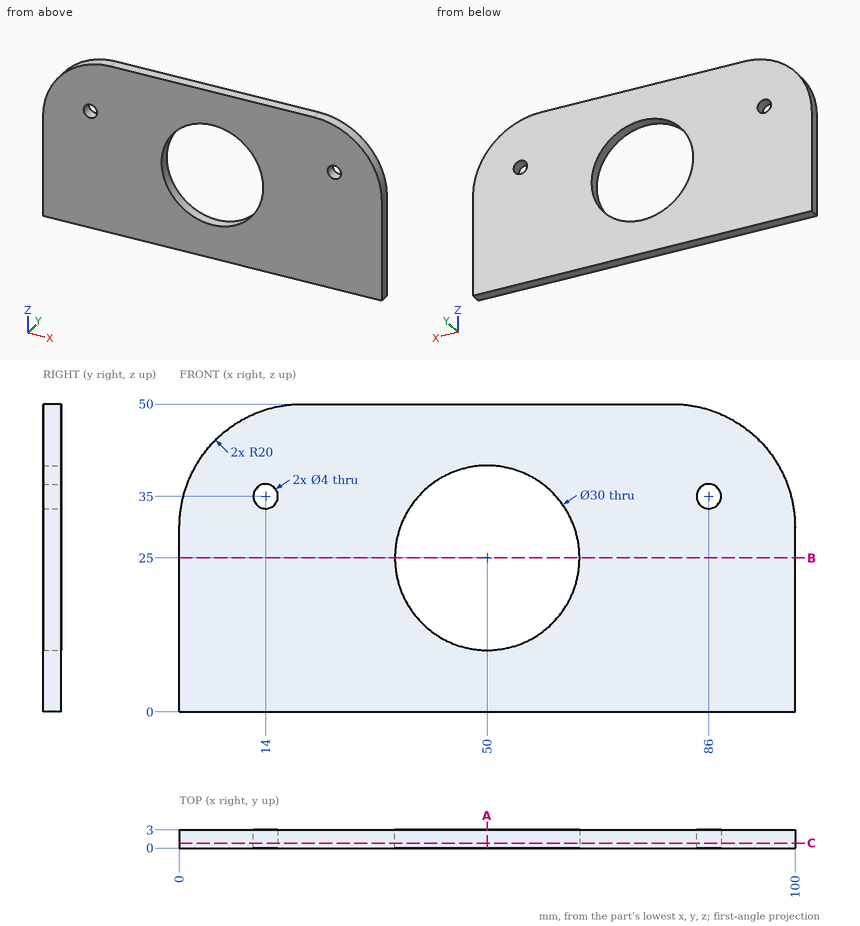
Source: three-view drawing plus pictorial views. Frame: mm from the lowest corner of the part. Round coordinates to 2 decimals unless told otherwise and drop trailing zeros. Order: outer loops, then holes, each group sorted by start corner. A loop starts at its lowest first (then second) coordinate and runs counter-clockwise, first axis right, second up. Notation, with made-up numbers: (-12.5, 33) - (8.5, 33) arc R22 ccw to (8.5, 58) - close; hole circle Ø4 at (-26.5, 72). An arc over 180 degrees is marked (long way). Write each question's results on one line, items separated by ' | '.
Item 1: First-contact query: pin 1 Ø2.5 at (x, z) = (86, 35) entering from -Y. Flat tip, straight axial feed; report the tip coordinate or a pass-through.
Completed:
pin 1: through
Item 2: Section B-B, the plane z = 25. Return the cut outline in (x, y), and give its area (3 significant figures).
Completed:
outline: (0, 0) - (35, 0) - (35, 3) - (0, 3) - close; (65, 0) - (100, 0) - (100, 3) - (65, 3) - close | area: 210 mm^2
Item 3: Section C-C, the plane y = 0.85. Return the cut outline in (x, z), and give its area (3 significant figures).
Completed:
outline: (0, 0) - (100, 0) - (100, 30) arc R20 ccw to (80, 50) - (20, 50) arc R20 ccw to (0, 30) - close; hole circle Ø4 at (14, 35); hole circle Ø30 at (50, 25); hole circle Ø4 at (86, 35) | area: 4,100 mm^2
Item 4: Section A-A, the plane x = 50. Return the cut outline in (y, z), and give its area (3 significant figures).
Completed:
outline: (0, 0) - (3, 0) - (3, 10) - (0, 10) - close; (0, 40) - (3, 40) - (3, 50) - (0, 50) - close | area: 60.0 mm^2
Item 5: Material intervals for line 1 along X through (y, z) = (1.3, 15.5); line 2 along Z through (x, y) = (50, 1.25); line 3 along Z through (x, y) = (54.5, 2.65), sorted ascending. Write a range as [from, to].
Completed:
line 1: [0, 38.39], [61.61, 100] | line 2: [0, 10], [40, 50] | line 3: [0, 10.69], [39.31, 50]
